Autodesk Inventor part; units mm, degrees
ref_plane "YZ Plane" through (0, 0, 0) normal (1, 0, 0) x (0, 1, 0)
ref_plane "XZ Plane" through (0, 0, 0) normal (0, 1, 0) x (-1, 0, 0)
ref_plane "XY Plane" through (0, 0, 0) normal (0, 0, 1) x (1, 0, 0)
sketch "Sketch1" plane through (0, 0, 0) normal (0, 1, 0) x (-1, 0, 0)
  line L0 (42.3333, 428.0371) -> (37.3333, 428.0371)
  line L1 (37.3333, 428.0371) -> (37.3333, 330.0371)
  line L2 (37.3333, 330.0371) -> (42.3333, 330.0371)
  line L3 (42.3333, 330.0371) -> (42.3333, 428.0371)
  point P0 (0, 0)
  dimension "d0" = 5
  dimension "d1" = 98
extrude "Extrusion1" add sketch "Sketch1" along normal blind 68
move or copy body "Move Body1" bodies to move or copy 1 copy no translate (15.875, -14.288, -387.35)
sketch "Sketch2" plane through (0, 68, 0) normal (0, 1, 0) x (1, 0, 0)
  line L0 (-26.4583, 57.3129) -> (-26.4583, -40.6871)
  line L1 (-21.4583, -40.6871) -> (-21.4583, 57.3129)
  line L2 (-26.4583, -15.6871) -> (-21.4583, -15.6871)
  line L3 (-21.4583, -15.6871) -> (-21.4583, -11.6871)
  line L4 (-21.4583, -11.6871) -> (-26.4583, -11.6871)
  line L5 (-26.4583, -11.6871) -> (-26.4583, -15.6871)
  line L6 (-26.4583, 28.3129) -> (-21.4583, 28.3129)
  line L7 (-21.4583, 28.3129) -> (-21.4583, 32.3129)
  line L8 (-21.4583, 32.3129) -> (-26.4583, 32.3129)
  line L9 (-26.4583, 32.3129) -> (-26.4583, 28.3129)
  line L10 (-26.4583, -40.6871) -> (-21.4583, -40.6871)
  line L11 (-21.4583, 57.3129) -> (-26.4583, 57.3129)
  line L12 (-21.4583, -40.6871) -> (-22.4583, -40.6871)
  line L13 (-22.4583, -40.6871) -> (-22.4583, 57.3129)
  line L14 (-22.4583, 57.3129) -> (-21.4583, 57.3129)
  line L15 (-21.4583, 57.3129) -> (-21.4583, -40.6871)
  point P0 (0, 0)
  point P1 (-26.4583, 32.3129)
  point P2 (-26.4583, 28.3129)
  point P3 (-26.4583, -11.6871)
  dimension "d7" = 29
  dimension "d8" = 29
  dimension "d9" = 25
  dimension "d10" = 25
  dimension "d26" = 1
move or copy body "Move Body2" bodies to move or copy 1 copy no translate (0, 14.288, 0)
extrude "Extrusion2" add sketch "Sketch2" along normal blind 6 contours L8 L13 L6 L0 | L8 L1 L6 L13 | L4 L13 L2 L0 | L4 L1 L2 L13
sketch "Sketch4" plane through (-26.4583, 68, 15.6871) normal (0, 0, 1) x (1, 0, 0)
  line L0 (0, 6) -> (5, 6)
  line L1 (5, 0) -> (5, 6)
  point P0 (26.4583, -68)
  point P1 (2.5, 3)
  dimension "d17" = 3
  dimension "d18" = 2.5
hole "Hole1" at (-23.9583, 71, 15.6871) direction (0, 0, -1) diameter 2.5 end through all
sketch "Sketch5" plane through (-21.4583, 0, 40.6871) normal (1, 0, 0) x (0, 0, -1)
  line L0 (40, 5) -> (58, 5)
  line L1 (58, 5) -> (58, 0)
  line L2 (58, 0) -> (40, 0)
  line L3 (40, 0) -> (40, 5)
  line L4 (0, 0) -> (98, 0)
  line L5 (0, 0) -> (0, 68)
  line L6 (98, 0) -> (98, 68)
  point P0 (40.6871, 0)
  dimension "d27" = 0
  dimension "d28" = 5
  dimension "d29" = 40
  dimension "d30" = 40
extrude "Extrusion3" add sketch "Sketch5" along normal blind 6
chamfer "Chamfer1" distance 4 angle 45 1 edges at (-15.4583, 5, -8.3129)
fillet "Fillet1" radius 2.5 4 edges at (-21.4583, 74, -30.3129) (-21.4583, 74, 13.6871) (-26.4583, 74, -30.3129) (-26.4583, 74, 13.6871)
properties part number "box_door"
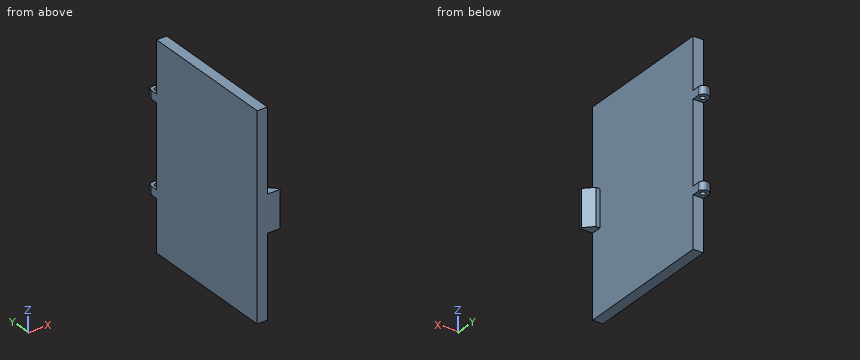
The model under review builds one solid part; all positions refer to its coordinate system, in mm. Round coordinates to 2 decimals unless told otherwise and drop trailing zeros. Loops run counter-clockwise (first coordinate to the right, second up) from the corner with the lowest first, then second, coordinate; pieces in that order, holes last. Notation, with made-up numbers: (48.5, 12.5) -> (84.5, 12.5) arc R19 cw to (84.5, 19.5) -> close; hole circle Ø3 at (-3, -12). An arc over 180 degrees is marked (long way). Answer as a JSON object with one key per item and string values. Group by question number.
1) We need section A-A on z = -6. Write out the cut boundary in (x, y).
2) We need section C-C on x = -17.5. Write out the cut boundary in (y, z), then the cut area to 3 significant figures.
3) We need section B-B on y = 61.5. Write out the cut boundary in (x, z).
4) For line 1 (X direction, y = 71, z = 14); line 2 (X direction, y = 40.5, z = 34.5); line 3 (Y direction, x = -24.25, z = 3), list the stretches that pass through material, from the lowest coordinate up. Write a range as [from, to].
5) For pin 1 Ø2 at (x, y) = (-23.96, 71) entering from -Z; pin 2 Ø5.5 at (x, y) = (-18, 2.5) entering from -Z; pin 3 Ø1.5 at (x, z) = (-25, -44.5) entering from +Y; pin 4 Ø1.5 at (x, y) = (-24.5, 72) entering from -Z, all flat-tipped, find the tip position at first contact; note any pin that passes through.
Result set:
{
 "1": {"outline": "(-26.46, 0) -> (-15.46, 0) -> (-15.46, 1) -> (-19.46, 5) -> (-21.46, 5) -> (-21.46, 68) -> (-26.46, 68) -> close"},
 "2": {"outline": "(0, -17.31) -> (3.04, -17.31) -> (3.04, 0.69) -> (0, 0.69) -> close", "area": "54.8 mm²"},
 "3": {"outline": "(-26.46, -57.31) -> (-21.46, -57.31) -> (-21.46, 40.69) -> (-26.46, 40.69) -> close"},
 "4": {"line 1": "[-26.46, -25.21], [-22.71, -21.46]", "line 2": "[-26.46, -21.46]", "line 3": "[0, 68]"},
 "5": {"pin 1": "through", "pin 2": "z = -17.31", "pin 3": "y = 68", "pin 4": "z = -32.31"}
}
